Design review of the part built by this model. Coordinates are the model's own, in mm. Round coordinates to 2 decimals unless told otherwise and drop trailing zeros. Loops run counter-clockwise (first coordinate to the right, second up) from the corner with the lowest first, then second, coordinate; pieces in that order, holes last. Notation, with made-up numbers: M -7,28 L 30,28 A13 ccw 30,33 Z; hole C 84.25,-8 d3. An arc over 180 degrees is marked long. One line per item, written item: value. Start each with the question number.
Item 1: For line 1 along X through (y, z) = (3.75, 172); line 2 along X through (y, z) = (-2.25, 320.5); line 3 along Z through (x, y) = (-36, 0), list the stretches that pass through material, from the lowest coordinate up.
Item 2: We need section B-B (y = 2.25). Write out the cut boundary in (x, z), then the cut area to 3 significant figures.
Item 3: Clearance check with a flat-ended pin moving along its axis: pin 1 (5 mm diameter, centred on x = 65.5, z = 450.5, fed in from +Y). State where the tip first meets the part, or that it passes through.
Item 4: We need section A-A (z = 624). Write out the cut boundary in (x, y).
from build123d import *

# Parameters (mm, degrees)
F0_W     = 150
F0_H     = 700
F1_DEPTH = 4.5
F3_DEPTH = 9.001
F5_DEPTH = 5


with BuildPart() as f1:
    # F0 (on Front) → F1 (new body, symmetric)
    with BuildSketch(Plane.XZ):
        with Locations((13.8296149671, 359)):
            Rectangle(F0_W, F0_H)
    extrude(amount=F1_DEPTH, both=True)

    # F2 (on face) → F3 (cut, through all)
    with BuildSketch(Plane.XZ.offset(4.5)):
        with BuildLine():
            ThreePointArc((-39.1703850329, 684), (-36.1703850329, 681), (-33.1703850329, 684))
            ThreePointArc((-33.1703850329, 684), (-36.1703850329, 687), (-39.1703850329, 684))
        make_face()
        with BuildLine():
            Line((-33.1703850329, 34), (-33.1703850329, 684))
            ThreePointArc((-33.1703850329, 684), (-36.1703850329, 681), (-39.1703850329, 684))
            Line((-39.1703850329, 684), (-39.1703850329, 34))
            ThreePointArc((-39.1703850329, 34), (-36.1703850329, 37), (-33.1703850329, 34))
        make_face()
        with BuildLine():
            ThreePointArc((-39.1703850329, 34), (-36.1703850329, 31), (-33.1703850329, 34))
            ThreePointArc((-33.1703850329, 34), (-36.1703850329, 37), (-39.1703850329, 34))
        make_face()
        with BuildLine():
            ThreePointArc((60.8296149671, 684), (63.8296149671, 681), (66.8296149671, 684))
            ThreePointArc((66.8296149671, 684), (63.8296149671, 687), (60.8296149671, 684))
        make_face()
        with BuildLine():
            Line((66.8296149671, 34), (66.8296149671, 684))
            ThreePointArc((66.8296149671, 684), (63.8296149671, 681), (60.8296149671, 684))
            Line((60.8296149671, 684), (60.8296149671, 34))
            ThreePointArc((60.8296149671, 34), (63.8296149671, 37), (66.8296149671, 34))
        make_face()
        with BuildLine():
            ThreePointArc((60.8296149671, 34), (63.8296149671, 31), (66.8296149671, 34))
            ThreePointArc((66.8296149671, 34), (63.8296149671, 37), (60.8296149671, 34))
        make_face()
    extrude(amount=-F3_DEPTH, mode=Mode.SUBTRACT)

    # F4 (on face) → F5 (cut)
    with BuildSketch(Plane(origin=(0, 4.5, 0), x_dir=(-1, 0, 0), z_dir=(0, 1, 0))):
        with BuildLine():
            Line((31.1703850329, 684), (31.1703850329, 34))
            ThreePointArc((31.1703850329, 34), (36.1703850329, 29), (41.1703850329, 34))
            Line((41.1703850329, 34), (41.1703850329, 684))
            ThreePointArc((41.1703850329, 684), (36.1703850329, 689), (31.1703850329, 684))
        make_face()
        with BuildLine():
            ThreePointArc((-68.8296149671, 34), (-63.8296149671, 29), (-58.8296149671, 34))
            Line((-58.8296149671, 34), (-58.8296149671, 684))
            ThreePointArc((-58.8296149671, 684), (-63.8296149671, 689), (-68.8296149671, 684))
            Line((-68.8296149671, 684), (-68.8296149671, 34))
        make_face()
    extrude(amount=-F5_DEPTH, mode=Mode.SUBTRACT)


solid = f1.part
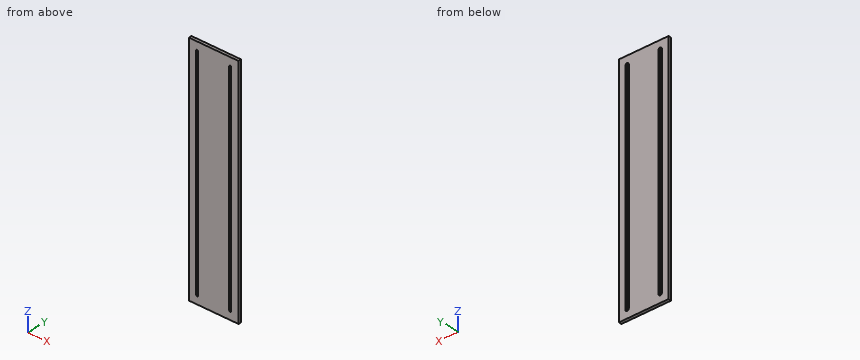
A:
1. line 1: -61.17 to -41.17, -31.17 to 58.83, 68.83 to 88.83
1. line 2: -61.17 to -39.17, -33.17 to 60.83, 66.83 to 88.83
1. line 3: 9 to 29, 689 to 709
2. outline: M -61.17,9 L 88.83,9 L 88.83,709 L -61.17,709 Z; hole M -41.17,34 A5 ccw -31.17,34 L -31.17,684 A5 ccw -41.17,684 Z; hole M 58.83,34 A5 ccw 68.83,34 L 68.83,684 A5 ccw 58.83,684 Z
2. area: 91,800 mm2
3. pin 1: y = -0.5
4. outline: M -61.17,-4.5 L -39.17,-4.5 L -39.17,-0.5 L -41.17,-0.5 L -41.17,4.5 L -61.17,4.5 Z; M -33.17,-4.5 L 60.83,-4.5 L 60.83,-0.5 L 58.83,-0.5 L 58.83,4.5 L -31.17,4.5 L -31.17,-0.5 L -33.17,-0.5 Z; M 66.83,-4.5 L 88.83,-4.5 L 88.83,4.5 L 68.83,4.5 L 68.83,-0.5 L 66.83,-0.5 Z
